Autodesk Inventor part; units mm, degrees
ref_plane "YZ Plane" through (0, 0, 0) normal (1, 0, 0) x (0, 1, 0)
ref_plane "XZ Plane" through (0, 0, 0) normal (0, 1, 0) x (-1, 0, 0)
ref_plane "XY Plane" through (0, 0, 0) normal (0, 0, 1) x (1, 0, 0)
sketch "Sketch1" plane through (0, 0, 0) normal (0, 1, 0) x (-1, 0, 0)
  line L0 (26.3596, 46.3409) -> (-11.7404, 46.3409)
  line L1 (-11.7404, 46.3409) -> (-11.7404, 20.9409)
  line L2 (-11.7404, 20.9409) -> (26.3596, 20.9409)
  line L3 (26.3596, 20.9409) -> (26.3596, 46.3409)
  point P0 (0, 0)
  dimension "d0" = 25.4
  dimension "d1" = 38.1
extrude "Extrusion1" add sketch "Sketch1" along normal blind 25.4
sketch "Sketch2" plane through (0, 25.4, 0) normal (0, 1, 0) x (1, 0, 0)
  line L0 (-26.3596, -46.3409) -> (11.7404, -46.3409)
  line L1 (-26.3596, -20.9409) -> (-26.3596, -46.3409)
  point P0 (0, 0)
  point P1 (-23.1846, -33.6409)
  point P2 (2.2154, -33.6409)
  dimension "d4" = 0
  dimension "d5" = 12.7
  dimension "d6" = 3.175
  dimension "d7" = 25.4
hole "Hole1" at (-23.1846, 25.4, 33.6409) at (2.2154, 25.4, 33.6409) direction (0, -1, 0) diameter 4.4958 end through all
sketch "Sketch3" plane through (-26.3596, 0, 46.3409) normal (0, 0, 1) x (1, 0, 0)
  line L0 (0, 0) -> (0, 25.4)
  line L1 (0, 25.4) -> (38.1, 25.4)
  point P0 (26.3596, 0)
  point P1 (12.7, 12.7)
  dimension "d15" = 12.7
  dimension "d16" = 12.7
hole "Hole2" at (-13.6596, 12.7, 46.3409) direction (0, 0, -1) diameter 6.35 end through all
properties part number "ElevDriveBlock"
Input: part model. Units: mm. Frame: model coordinates. Round coordinates to 2 decimals unless told otherwise and drop trailing zeros. Order: outer loops, then holes, each group sorted by start corner. A loop starts at its lowest first (then second) coordinate and runs counter-clockwise, first axis right, second up. Notation, with made-up numbers: (0.5, 2) - (40.5, 2) arc R22 ccw to (40.5, 12) - close; hole circle Ø8 at (52, 45). An arc over 180 degrees is marked (long way). Use a Markdown table: item, result.
1. Section B-B on x = 3.5. Return the cut outline in (y, z), then the cut area to 3 significant figures.
Evaluation:
| item | result |
|---|---|
| outline | (0, 20.94) - (25.4, 20.94) - (25.4, 31.8) - (0, 31.8) - close; (0, 35.49) - (25.4, 35.49) - (25.4, 46.34) - (0, 46.34) - close |
| area | 551 mm^2 |
2. Section C-C on y = 3. Return the cut outline in (x, z), then the cut area to 3 significant figures.
Evaluation:
| item | result |
|---|---|
| outline | (-26.36, 20.94) - (11.74, 20.94) - (11.74, 46.34) - (-26.36, 46.34) - close; hole circle Ø4.5 at (-23.18, 33.64); hole circle Ø4.5 at (2.22, 33.64) |
| area | 936 mm^2 |
3. Section D-D on z = 23. Return the cut outline in (x, y) (3 decimals), then the cut area to 3 significant figures.
Evaluation:
| item | result |
|---|---|
| outline | (-26.36, 0) - (11.74, 0) - (11.74, 25.4) - (-26.36, 25.4) - close; hole circle Ø6.35 at (-13.66, 12.7) |
| area | 936 mm^2 |
4. Section A-A on y = 12.7. Return the cut outline in (x, z), then the cut area to 3 significant figures.
Evaluation:
| item | result |
|---|---|
| outline | (-26.36, 20.94) - (-16.83, 20.94) - (-16.83, 46.34) - (-26.36, 46.34) - close; (-10.48, 20.94) - (11.74, 20.94) - (11.74, 46.34) - (-10.48, 46.34) - close; hole circle Ø4.5 at (-23.18, 33.64); hole circle Ø4.5 at (2.22, 33.64) |
| area | 775 mm^2 |
5. Mould query, pull axis X, two halves, no side actions, for faces 1 (the face through (-26.36, 13, 33)), 2 (the face through (3.076, 12.522, 35.717)), 3 (the face through (-7, 25.4, 34)), 4 (the face through (-25.08, 12.52, 34.85)). Classes: +X half, -X half, draft (parallel to the pull), parting line (faces both ways), or undercut.
Evaluation:
| item | result |
|---|---|
| face 1 | -X half |
| face 2 | undercut |
| face 3 | draft |
| face 4 | undercut |
6. Material intervals for probe 1 along X at (y, z) = (21, 33.5); probe 2 along X at (y, z) = (12.75, 37.25) (3 decimals); probe 3 along Y at (x, z) = (-13.5, 43.5), sorted ascending.
Evaluation:
| item | result |
|---|---|
| probe 1 | -26.36 to -25.43, -20.94 to -0.03, 4.46 to 11.74 |
| probe 2 | -26.36 to -16.834, -10.485 to 11.74 |
| probe 3 | 0 to 9.53, 15.87 to 25.4 |
